Check sheet for the modelled part. Datum: model origin and axes. Units: mm. A direction names the side the tool comes from. Coordinates: 2 decimals unless noted, no trailing zeros. Loops run counter-clockwise (first coordinate to the right, second up) from the corner with the lowest first, then second, coordinate; pieces in that order, holes last. Notation, with made-up numbers: (1.25, -25.75) - (44.25, -25.75) arc R29 cw to (44.25, 9.25) - close; hole circle Ø2 at (9, 16). An arc over 180 degrees is marked (long way). Use a Markdown table: item, result. Add a question column.
1) Sectioned sample at B-B, the plane y = -55. Enter the section's corners in (x, z).
2) Sectioned sample at A-A, the plane x = 0. Enter the section's corners in (y, z).
3) Sectioned sample at D-D, the plane y = 3. Enter the section's corners in (x, z), then the cut area to 3 significant figures.
4) Thickness scan on line 1 (Y direction, x = -16, z = 100); line 2 (Y direction, x = 0, z = 14.75); line 3 (X direction, y = 55, z = 15). Record the ranges inside material, lowest first.
5) Draft check along Z on faces 3 (the flat face through (-20, 2, 13)), 4 (the flat face through (-10, -6, 100)), 5 (the flat face through (0, 1, 0)). Enter one of: pulls with the +Z half, pulls with the -Z half, needs draft (parallel to the pull), parting line crosses it, or undercut.
6) Sectioned sample at C-C, the plane x = -13.5. Enter the section's corners in (y, z), then the cut area to 3 significant figures.
7) Tool access check on faces 1 (the cylindrical face through (-14.93, -6.751, 102.385)), 2 (the cylindrical face through (0.867, 51.095, 12.878)). Record the directions out of +Z, -Z, +X, -X, +Y, -Y that give a thin tool (end or side, any length) a straight path to the whole face; none if there is none.
8) Go/stop test with flat-tipped pins: P1, Ø3, axis at x = -14.5, z = 20, coming from the -Y side; P2, Ø3, axis at y = -6, z = 100, coming from the -X side; P3, Ø5, axis at x = 1, y = -39, coming from the -Z side; P4, Ø2, axis at x = -4, z = 70, coming from the -Y side. Record where each tip stops, or that it passes through.
Autodesk Inventor part; units mm, degrees
ref_plane "YZ Plane" through (0, 0, 0) normal (1, 0, 0) x (0, 1, 0)
ref_plane "XZ Plane" through (0, 0, 0) normal (0, 1, 0) x (-1, 0, 0)
ref_plane "XY Plane" through (0, 0, 0) normal (0, 0, 1) x (1, 0, 0)
sketch "Sketch1" plane through (0, 0, 0) normal (1, 0, 0) x (0, 1, 0)
  line L0 (0, 144) -> (0, -24) construction
  line L1 (-138.8268, 0) -> (138.8268, 0) construction
  line L2 (-62.5, 0) -> (-62.5, 18.8952)
  line L3 (62.5, 0) -> (62.5, 18.8952)
  line L4 (25, 120) -> (-25, 120)
  line L5 (62.5, 0) -> (-62.5, 0)
  arc A0 (25, 120) -> (62.5, 18.8952) centre (99.162, 90) ccw
  arc A1 (-62.5, 18.8952) -> (-25, 120) centre (-99.162, 90) ccw
  point P0 (0, 0)
  dimension "d0" = 120
  dimension "d1" = 125
  dimension "d3" = 50
  dimension "d4" = 80
  dimension "d6" = 90
extrude "Main Body" add sketch "Sketch1" along normal mid plane 20
sketch "Sketch2" plane through (10, 62.5, 0) normal (0, 0, -1) x (-1, 0, 0)
  line L0 (20, 0) -> (0, 0)
  line L1 (10, 0) -> (10, -125) construction
  line L2 (20, -125) -> (0, -125)
  line L3 (0, -37.5) -> (0, -87.5)
  line L4 (0, -62.5) -> (20, -62.5) construction
  line L5 (20, -87.5) -> (20, -37.5)
  circle A0 centre (10, -7.5) radius 4
  circle A1 centre (10, -117.5) radius 4
  point P0 (10, -62.5)
  dimension "d9" = 110
  dimension "d10" = 8
extrude "Upright Mount Holes" cut sketch "Sketch2" against normal through all
sketch "Sketch3" plane through (-10, 0, 0) normal (-1, 0, 0) x (0, 0, 1)
  line L0 (0, 87.5) -> (0, -87.5) construction
  line L1 (-24, 0) -> (144, 0) construction
  circle A0 centre (15.4778, 3) radius 5
  circle A1 centre (100, -6) radius 5
  line L2 (15.4778, 3) -> (100, -6) construction
  circle A2 centre (15.4778, 3) radius 2.5
  circle A3 centre (100, -6) radius 2.5
  point P0 (0, 0)
  dimension "d13" = 6
  dimension "d14" = 3
  dimension "d15" = 100
  dimension "d16" = 85
  dimension "d17" = 10
  dimension "d18" = 5
extrude "Extrusion3" add sketch "Sketch3" along normal blind 10
properties part number "Caliper Bracket Mount V2"
Solved:
| question | item | result |
|---|---|---|
| 1 | outline | (-10, 0) - (-4, 0) - (-4, 23.29) - (-10, 23.29) - close; (4, 0) - (10, 0) - (10, 23.29) - (4, 23.29) - close |
| 2 | outline | (-62.5, 0) - (-59, 0) - (-59, 20.81) arc R80 cw to (-62.5, 18.9) - close; (-51, 0) - (51, 0) - (51, 26.12) arc R80 cw to (25, 120) - (-25, 120) arc R80 cw to (-51, 26.12) - close; (59, 0) - (62.5, 0) - (62.5, 18.9) arc R80 cw to (59, 20.81) - close |
| 3 | outline | (-20, 10.48) - (-10, 10.48) - (-10, 0) - (10, 0) - (10, 120) - (-10, 120) - (-10, 20.48) - (-20, 20.48) - (-20, 17.98) - (-10, 17.98) - (-10, 12.98) - (-20, 12.98) - close |
| 3 | area | 2,450 mm2 |
| 4 | line 1 | y = -11 to -8.5, -3.5 to -1 |
| 4 | line 2 | y = -62.5 to -59, -51 to 51, 59 to 62.5 |
| 4 | line 3 | x = -10 to -4, 4 to 10 |
| 5 | face 3 | needs draft |
| 5 | face 4 | undercut |
| 5 | face 5 | pulls with the -Z half |
| 6 | outline | circle Ø10 at (-6, 100); circle Ø10 at (3, 15.48); hole circle Ø5 at (-6, 100); hole circle Ø5 at (3, 15.48) |
| 6 | area | 118 mm2 |
| 7 | face 1 | -X |
| 7 | face 2 | +Z, -Z |
| 8 | P1 | stops at y = -0.98 |
| 8 | P2 | stops at x = -10 |
| 8 | P3 | stops at z = 0 |
| 8 | P4 | stops at y = -21.97 |
